Here's the drawing with two shaded views (mm, measured from the low corner). I have some questions. Round coordinates to 2 decimals unless told otherwise and drop trailing zeros. Loops run counter-clockwise (first coordinate to the right, second up) from the corner with the lowest first, then second, coordinate; pieces in that order, holes last.
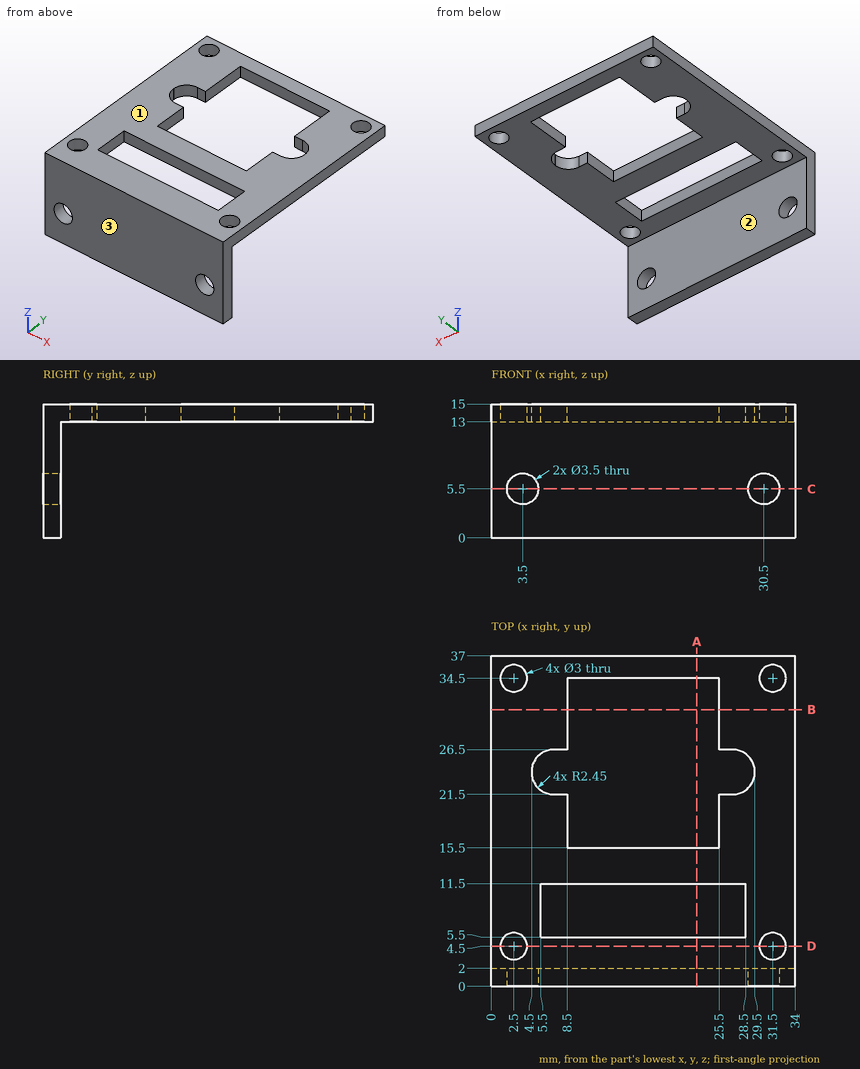
(1) If we section it at D-D, the plane y = 4.5: List the corners of the cut face in (x, z) for me.
Worked answers:
outline: (0, 13) - (1, 13) - (1, 15) - (0, 15) - close; (4, 13) - (30, 13) - (30, 15) - (4, 15) - close; (33, 13) - (34, 13) - (34, 15) - (33, 15) - close
(2) If we section it at A-A, the plane x = 23: List the corners of the cut face in (y, z) for me, then the cut area to 3 significant figures.
Worked answers:
outline: (0, 0) - (2, 0) - (2, 13) - (5.5, 13) - (5.5, 15) - (0, 15) - close; (11.5, 13) - (15.5, 13) - (15.5, 15) - (11.5, 15) - close; (34.5, 13) - (37, 13) - (37, 15) - (34.5, 15) - close
area: 50.0 mm2
(3) If I drill on line 1 (Y direction, x = 31.5, z = 14); line 2 (X direction, y = 1.4, z = 5.5); line 3 (Y direction, x = 8, z = 14.25), over which ranges is the centre line in solid material (lowest first)?
Worked answers:
line 1: y = 0 to 3, 6 to 33, 36 to 37
line 2: x = 0 to 1.75, 5.25 to 28.75, 32.25 to 34
line 3: y = 0 to 5.5, 11.5 to 21.5, 26.5 to 37
(4) If we mould it in two halves opening along Y, with no side actions, what happens to the marked faces 1, 2 and 3? For each: released by +Y, released by -Y, zero draft, split by the parting line, or undercut.
Worked answers:
face 1: zero draft
face 2: released by +Y
face 3: released by -Y
(5) If we section it at C-C, the plane z = 5.5: List the corners of the cut face in (x, y) for me.
Worked answers:
outline: (0, 0) - (1.75, 0) - (1.75, 2) - (0, 2) - close; (5.25, 0) - (28.75, 0) - (28.75, 2) - (5.25, 2) - close; (32.25, 0) - (34, 0) - (34, 2) - (32.25, 2) - close
(6) Will this pin go through, and if not, where does the flat tip stop? P1, Ø3, axis at x = 15.5, y = 8, coming from the +Z side.
Worked answers:
P1: passes through
(7) If we section it at B-B, the plane y = 31: List the corners of the cut face in (x, z) for me, then the cut area to 3 significant figures.
Worked answers:
outline: (0, 13) - (8.5, 13) - (8.5, 15) - (0, 15) - close; (25.5, 13) - (34, 13) - (34, 15) - (25.5, 15) - close
area: 34.0 mm2
